Source: CAD feature listing. Evaluate the final solid. Frame: model axes, mm. Round coordinates to 2 decimals unless told otherwise and drop trailing zeros. Loops run counter-clockwise (first coordinate to the right, second up) from the corner with the lowest first, then second, coordinate; pieces in that order, holes last. Notation, with made-up numbers: (-9.75, 9.5) - (0.25, 9.5) arc R9 ccw to (0.25, 18.5) - close; hole circle Ø3 at (65.25, 73.5). An arc over 180 degrees is marked (long way). Write item = value, one per line. Start each with the question number.
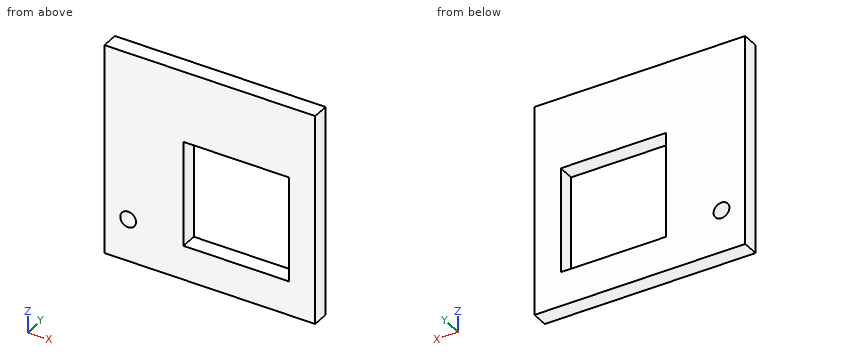
from build123d import *

# Parameters (mm, degrees)
F0_W     = 80
F0_H     = 80
F1_DEPTH = 6.35
F2_W     = 40
F2_H     = 40
F2_R     = 3
F3_DEPTH = 6.351


with BuildPart() as f1:
    # F0 (on Front) → F1 (new body)
    with BuildSketch(Plane.XZ):
        Rectangle(F0_W, F0_H)
    extrude(amount=F1_DEPTH)

    # F2 (on face) → F3 (cut, through all)
    with BuildSketch(Plane.XZ.offset(6.35)):
        with Locations((10, -7)):
            Rectangle(F2_W, F2_H)
        with Locations((-31, -24)):
            Circle(F2_R)
    extrude(amount=-F3_DEPTH, mode=Mode.SUBTRACT)


solid = f1.part
(1) Material intervals for line 1 along X through (y, z) = (-4.5, -4.5); line 2 along Z through (x, y) = (-31, -4); line 3 along Z through (x, y) = (22.5, -5.5), sorted ascending. Write a range as from..to.
(2) Cut plane D-D (z = -3). Output: boundary loops of the cut face in (x, y), and give its area (3 significant figures).
(3) Cut plane B-B (x = 1.5). Output: boundary loops of the cut face in (y, z), and give its area (3 significant figures).
(4) Pin query (flat end, axial travel): P1, Ø3.5, axis at x = -31, z = -24, coming from the -Y side. Return the tip coordinate at first contact, or that it passes through.
(5) Cut plane A-A (z = -24). Output: boundary loops of the cut face in (x, y), and give its area (3 significant figures).
(6) Cut plane C-C (y = -2). Output: boundary loops of the cut face in (x, z).
Solution:
q1.line_1 = -40..-10, 30..40
q1.line_2 = -40..-27, -21..40
q1.line_3 = -40..-27, 13..40
q2.outline = (-40, -6.35) - (-10, -6.35) - (-10, 0) - (-40, 0) - close; (30, -6.35) - (40, -6.35) - (40, 0) - (30, 0) - close
q2.area = 254 mm^2
q3.outline = (-6.35, -40) - (0, -40) - (0, -27) - (-6.35, -27) - close; (-6.35, 13) - (0, 13) - (0, 40) - (-6.35, 40) - close
q3.area = 254 mm^2
q4.P1 = through
q5.outline = (-40, -6.35) - (-34, -6.35) - (-34, 0) - (-40, 0) - close; (-28, -6.35) - (-10, -6.35) - (-10, 0) - (-28, 0) - close; (30, -6.35) - (40, -6.35) - (40, 0) - (30, 0) - close
q5.area = 216 mm^2
q6.outline = (-40, -40) - (40, -40) - (40, 40) - (-40, 40) - close; hole circle Ø6 at (-31, -24); hole (-10, -27) - (30, -27) - (30, 13) - (-10, 13) - close
